```python
from build123d import *

# Parameters (mm, degrees)
CUT_EXTRUDE1_DEPTH         = 58.529738397
CUT_EXTRUDE1_DEPTH_BACK    = 58.529738397
F_1_4_28_TAPPED_HOLE1_D    = 5.4102
CUT_EXTRUDE2_START         = -6.35
SKETCH5_R                  = 30.48
CUT_EXTRUDE2_DEPTH         = 6.35
USE_ROUND_CORNER_ENDMILL_R = 0.762
F_1_4_CLEARANCE_HOLE1_D    = 6.5278


with BuildPart() as part:
    # MASTER → MASTER_SKETCH (revolve)
    with BuildSketch(Plane.XY):
        Polygon((0, 38.1), (-30.48, 38.1), (-30.48, 0), (-12.7, 0), (-12.7, 19.05), (-6.3246, 19.05), (-4.7625, 17.4879), (0, 17.4879), align=None)
    revolve(axis=Axis((0, 38.1, 0), (0, -1, 0)))

    # Sketch2 → Cut-Extrude1 (cut, two sides: drawn at the far end of the back side and taken through both)
    with BuildSketch(Plane.XY.offset(-CUT_EXTRUDE1_DEPTH_BACK)):
        Polygon((-30.48, 20.248277745), (-9.205145869, 38.1), (-30.48, 38.1), align=None)
        Polygon((30.48, 38.1), (9.205145869, 38.1), (30.48, 20.248277745), align=None)
    extrude(amount=CUT_EXTRUDE1_DEPTH + CUT_EXTRUDE1_DEPTH_BACK, mode=Mode.SUBTRACT)

    # 1/4-28 Tapped Hole1 (through all)
    with Locations(Plane(origin=(0, 38.1, 0), x_dir=(1, 0, 0), z_dir=(0, 1, 0))):
        with Locations((0, 0)):
            Hole(F_1_4_28_TAPPED_HOLE1_D / 2)

    # Sketch5 → Cut-Extrude2 (cut)
    with BuildSketch(Plane(origin=(0, 38.1, 0), x_dir=(1, 0, 0), z_dir=(0, 1, 0)).offset(CUT_EXTRUDE2_START)):
        with Locations(Location((0, 0, 0), (0, 0, 180))):
            Circle(SKETCH5_R)
    extrude(amount=CUT_EXTRUDE2_DEPTH, mode=Mode.SUBTRACT)

    # use-round-corner-endmill
    use_round_corner_endmill_edges = [part.edges().sort_by_distance(p)[0] for p in [
        (6.3246, 19.05, 0),
        (12.7, 19.05, 0),
    ]]
    fillet(use_round_corner_endmill_edges, radius=USE_ROUND_CORNER_ENDMILL_R)

    # Sketch7 → 1/4 NPT Tapped Hole1 (revolve, cut)
    with BuildSketch(Plane(origin=(-23.455832083, 26.142254454, 0), x_dir=(-0.7660444431189741, -0.642787609686544, 0), z_dir=(0, 0, 1))):
        Polygon((0, 0), (0, 54.695413336), (5.5626, 54.695413336), (5.5626, 9.906), (6.557984794, 9.906), (6.8545837, 0), align=None)
    f_1_4_npt_tapped_hole1 = revolve(axis=Axis((-27.537533405, 31.006636667, 0), (0.6427876096865441, -0.7660444431189741, 0)), mode=Mode.SUBTRACT)

    # Mirror1: 1/4 NPT Tapped Hole1 across plane
    add(f_1_4_npt_tapped_hole1.mirror(Plane(origin=(0, 0, 0), x_dir=(0, 0, 1), z_dir=(1, 0, 0))), mode=Mode.SUBTRACT)

    # 1/4 Clearance Hole1 (through all)
    with Locations(Plane(origin=(0, 31.75, 0), x_dir=(1, 0, 0), z_dir=(0, 1, 0))):
        with Locations((-12.7, -21.997045256), (12.7, -21.997045256), (12.7, 21.997045256), (-12.7, 21.997045256)):
            Hole(F_1_4_CLEARANCE_HOLE1_D / 2)


solid = part.part
```
Design review of the part built by this model. Coordinates are the model's own, in mm. A direction names the side the tool comes from. Give positions to 0.01 mm unless a question says otherwise; leave off trailing zeros. Write each loop counter-clockwise with the first axis right and the second up, starting at its lowest first coordinate (ties: lowest second). Pieces come first, ordered by that corner, then holes. Notation, with made-up numbers: (-1.75, -25) -> (48.25, -25) arc R30 ccw to (48.25, 1) -> close; hole circle Ø2 at (-11.75, -14). An arc over 180 degrees is marked (long way). Answer in a Markdown table with one row per item.
(1) Consider section A-A (x = 0). State the section outline as (y, z) points.
Results:
| item | result |
|---|---|
| outline | (0, -30.48) -> (31.75, -30.48) -> (31.75, -2.71) -> (17.49, -2.71) -> (17.49, -4.76) -> (18.83, -6.1) arc R0.76 cw to (19.05, -6.64) -> (19.05, -11.94) arc R0.76 cw to (18.29, -12.7) -> (0, -12.7) -> close; (0, 12.7) -> (18.29, 12.7) arc R0.76 cw to (19.05, 11.94) -> (19.05, 6.64) arc R0.76 cw to (18.83, 6.1) -> (17.49, 4.76) -> (17.49, 2.71) -> (31.75, 2.71) -> (31.75, 30.48) -> (0, 30.48) -> close |
(2) To check wall thickness, follow probe 1 along Z at (x, y) = (-13.5, 28); probe 2 along Z at (x, y) = (-14, 23); probe 3 along Z at (x, y) = (12, 9) (3 decimals). State the ranges of each line that lie inside material, in increasing order.
Results:
| item | result |
|---|---|
| probe 1 | -27.33 to -25.16, -18.83 to 18.83, 25.16 to 27.33 |
| probe 2 | -27.07 to -24.99, -19 to -4.03, 4.03 to 19, 24.99 to 27.07 |
| probe 3 | -28.018 to -25.185, -18.809 to -5.09, 5.09 to 18.809, 25.185 to 28.018 |
(3) Consider section B-B (z = 0). Count the separate pieces of the cut face and the enclosed holes in it, then the cut area to 3 significant figures.
Results:
| item | result |
|---|---|
| separate pieces | 4 |
| enclosed holes | 0 |
| area | 809 mm2 |
(4) Clearance check with flat-ended pins moving along their axes: pin 1 (5 mm diameter, centred on x = 1.5, z = 1.5, fed in from -Y); pin 2 (5 mm diameter, centred on x = -12.7, z = -22, fed in from -Y); pin 3 (2 mm diameter, centred on x = -22.5, y = 8, fed in from -Z); pin 4 (1 mm diameter, centred on x = -13, y = 6.5, fed in from +Z). State where each tip first meets the part, or that it passes through.
Results:
| item | result |
|---|---|
| pin 1 | y = 17.49 |
| pin 2 | through |
| pin 3 | z = -21.61 |
| pin 4 | z = 27.8 |
(5) Mouldability with a two-part tool opening along Z and no side actions: class faces 1 (the flat face through (-2.05, 17.488, 2.05)), 2 (the flat face through (-17.63, 31.03, -0.36)), 3 (the conical face through (25.064, 18.418, 2.569)), 4 (the cylindrical face through (3.97, 12.12, -30.22)) as +Z half, -Z half, draft (parallel to the pull), parting line (faces both ways), or undercut.
Results:
| item | result |
|---|---|
| face 1 | undercut |
| face 2 | draft |
| face 3 | undercut |
| face 4 | parting line |
(6) Consider section C-C (y = 3.5). State the section outline as (x, z) points, then the cut area to 3 significant figures.
Results:
| item | result |
|---|---|
| outline | circle Ø60.96 at (0, 0); hole circle Ø6.53 at (-12.7, -22); hole circle Ø6.53 at (-12.7, 22); hole circle Ø25.4 at (0, 0); hole circle Ø6.53 at (12.7, -22); hole circle Ø6.53 at (12.7, 22) |
| area | 2,280 mm2 |
(7) For faces 5 (the flat face through (-5, 19.05, 5)), 6 (the cylindrical face through (-10.11, 15.65, -20.01)), list the 3-axis set-ups (+Z, -Z, +X, -X, +Y, -Y) from which the entire face can be reached by the end or side of a thin tool; tool diameter is ignored.
Results:
| item | result |
|---|---|
| face 5 | -Y |
| face 6 | +Y, -Y |
